Source: CAD feature listing. Evaluate the final solid. Frame: model axes, mm. A direction names the side the tool comes from. Round coordinates to 2 decimals unless told otherwise and drop trailing zeros. Order: outer loops, then holes, each group sorted by start corner. A loop starts at its lowest first (then second) coordinate and runs counter-clockwise, first axis right, second up. Notation, with made-up numbers: M 48.25,71 L 53.25,71 A34 ccw 53.25,102 Z; hole C -7.5,34 d6. An arc over 180 degrees is marked long. Use one line per item in the form item = value. Start each with the question number.
Q1. Section C-C (z = 27.5). Return the cut outline in (x, y), plus the area to 3 significant figures.
Q2. Section A-A (x = -34). Return the cut outline in (y, z).
Q3. Pull-direction query (Y, two-part tool) for faces 4 (the flat face through (19, 0, 19)), 5 (the flat face through (13, 6.35, -29.4)), 6 (the cylindrical face through (16.55, 3.13, -31.96)); classes: pulls with the +Y half, pulls with the -Y half, needs draft (parallel to the pull), parting line crosses it, or undercut.
Q4. Section B-B (x = 38.1). Return the cut outline in (y, z).
Q5. Contact query for flat-ended pins moving along their axis: pin 1 (3 mm diameter, centred on x = 0, z = 38.1, fed in from -Y); pin 2 (6 mm diameter, centred on x = 33, z = -19.05, fed in from +Y); pin 3 (1.5 mm diameter, centred on x = 18, z = 15.5, fed in from -Y); pin 4 (2 mm diameter, centred on y = 60, z = -12.5, fed in from -X). Output: stop coordinate, or through.
Q6. Material intervals for probe 1 along Y at (x, z) = (16, -28.5); probe 2 along Z at (x, y) = (0, 110); probe 3 along X at (y, z) = (4.25, -19.05), sorted ascending.
Q7. Reachability of faces 1 (the cylindrical face through (30.415, 3.131, 18.237)), 2 (the cylindrical face through (30.995, 61.081, 6.883)), 3 (the cylindrical face through (24.796, 107.739, 5.506)) from +Z, -Z, +X, -X, +Y, -Y: full face, straight path, thin tool, end or side. Return the list, or none.
Q8. Section D-D (y = 29). Return the cut outline in (x, z).
from build123d import *

# Parameters (mm, degrees)
F_3_0_213_DIAMETER_HOLE3_D = 5.4102


with BuildPart() as part:
    # Sketch1 → Chamber (revolve)
    with BuildSketch(Plane(origin=(0, 0, 0), x_dir=(0, 0, -1), z_dir=(1, 0, 0))):
        Polygon((31.75, 6.35), (31.75, 114.3), (44.45, 114.3), (44.45, 120.65), (31.75, 120.65), (25.4, 120.65), (25.4, 114.3), (25.4, 6.35), (25.4, 0), (31.75, 0), (44.45, 0), (44.45, 6.35), align=None)
    revolve(axis=Axis((0, 0, 0), (0, 1, 0)))

    # Sketch4 → Turbulence Rings (revolve)
    with BuildSketch(Plane(origin=(0, 0, 0), x_dir=(0, 0, -1), z_dir=(1, 0, 0))):
        Polygon((25.4, 92.643708368), (25.4, 95.183708368), (7.62, 77.403708368), (7.62, 74.863708368), align=None)
    revolve(axis=Axis((0, 0, 0), (0, 1, 0)))

    # #3 (0.213) Diameter Hole3 (through all)
    with Locations(Plane(origin=(0, 120.65, 0), x_dir=(1, 0, 0), z_dir=(0, 1, 0))):
        with Locations((0, 0), (-38.1, 0), (-32.995567884, 19.05), (-19.05, 32.995567884), (0, 38.1), (19.05, 32.995567884), (32.995567884, 19.05), (38.1, 0), (32.995567884, -19.05), (19.05, -32.995567884), (0, -38.1), (-19.05, -32.995567884), (-32.995567884, -19.05)):
            Hole(F_3_0_213_DIAMETER_HOLE3_D / 2)


solid = part.part
Results list:
q1.outline = M -34.92,0 L 34.92,0 L 34.92,6.35 L 15.87,6.35 L 15.87,114.3 L 34.92,114.3 L 34.92,120.65 L -34.92,120.65 L -34.92,114.3 L -15.87,114.3 L -15.87,6.35 L -34.92,6.35 Z
q1.area = 4,310 mm2
q2.outline = M 0,-28.63 L 6.35,-28.63 L 6.35,-21.56 L 0,-21.56 Z; M 0,-16.54 L 6.35,-16.54 L 6.35,16.54 L 0,16.54 Z; M 0,21.56 L 6.35,21.56 L 6.35,28.63 L 0,28.63 Z; M 114.3,-28.63 L 120.65,-28.63 L 120.65,-21.56 L 114.3,-21.56 Z; M 114.3,-16.54 L 120.65,-16.54 L 120.65,16.54 L 114.3,16.54 Z; M 114.3,21.56 L 120.65,21.56 L 120.65,28.63 L 114.3,28.63 Z
q3.face_4 = pulls with the -Y half
q3.face_5 = undercut
q3.face_6 = needs draft
q4.outline = M 0,-22.9 L 6.35,-22.9 L 6.35,-2.71 L 0,-2.71 Z; M 0,2.71 L 6.35,2.71 L 6.35,22.9 L 0,22.9 Z; M 114.3,-22.9 L 120.65,-22.9 L 120.65,-2.71 L 114.3,-2.71 Z; M 114.3,2.71 L 120.65,2.71 L 120.65,22.9 L 114.3,22.9 Z
q5.pin_1 = through
q5.pin_2 = 120.65
q5.pin_3 = 90.25
q5.pin_4 = -29.59
q6.probe_1 = 0 to 6.35, 114.3 to 120.65
q6.probe_2 = -31.75 to -25.4, 25.4 to 31.75
q6.probe_3 = -40.16 to -35.7, -30.29 to -16.8, 16.8 to 30.29, 35.7 to 40.16
q7.face_1 = +Y, -Y
q7.face_2 = none
q7.face_3 = +Y
q8.outline = C 0,0 d63.5; hole C 0,0 d50.8
